from build123d import *

# Parameters (mm, degrees)
ESQUISSE1_W        = 45
ESQUISSE1_H        = 36
BOSS_EXTRU_1_DEPTH = 8
ESQUISSE2_W        = 10.16
ESQUISSE2_H        = 7.62
BOSS_EXTRU_2_DEPTH = 6
ESQUISSE3_R        = 1
BOSS_EXTRU_3_DEPTH = 15
ESQUISSE4_R        = 1
BOSS_EXTRU_4_DEPTH = 15


with BuildPart() as part:
    # Esquisse1 → Boss.-Extru.1 (new body)
    with BuildSketch(Plane(origin=(0, 0, 0), x_dir=(1, 0, 0), z_dir=(0, 1, 0))):
        Rectangle(ESQUISSE1_W, ESQUISSE1_H)
    extrude(amount=BOSS_EXTRU_1_DEPTH)

    # Esquisse2 → Boss.-Extru.2 (add)
    with BuildSketch(Plane.ZY.offset(22.5)):
        with Locations((6.482241764, 4)):
            Rectangle(ESQUISSE2_W, ESQUISSE2_H)
    extrude(amount=BOSS_EXTRU_2_DEPTH)

    # Esquisse3 → Boss.-Extru.3 (add)
    with BuildSketch(Plane.ZY.offset(22.5)):
        with Locations(Location((15.846041743, 6, 0), (0, 0, 180))):
            Circle(ESQUISSE3_R)
        with Locations(Location((15.846041743, 2, 0), (0, 0, 180))):
            Circle(ESQUISSE3_R)
    extrude(amount=BOSS_EXTRU_3_DEPTH)

    # Esquisse4 → Boss.-Extru.4 (add)
    with BuildSketch(Plane(origin=(22.5, 0, 0), x_dir=(0, 0, -1), z_dir=(1, 0, 0))):
        with Locations(Location((-16.5, 5.5, 0), (0, 0, 180))):
            Circle(ESQUISSE4_R)
        with Locations(Location((-16.5, 2.5, 0), (0, 0, 180))):
            Circle(ESQUISSE4_R)
        with Locations(Location((-13.5, 2.5, 0), (0, 0, 180))):
            Circle(ESQUISSE4_R)
        with Locations(Location((-13.5, 5.5, 0), (0, 0, 180))):
            Circle(ESQUISSE4_R)
    extrude(amount=BOSS_EXTRU_4_DEPTH)


solid = part.part
Can you work these out from the model? Positions are in its coordinate system, mm. A direction names the side the tool comes from. Give positions to 0.01 mm unless a question says otherwise; leave off trailing zeros. Loops run counter-clockwise (first coordinate to the right, second up) from the corner with the lowest first, then second, coordinate; pieces in that order, holes last. Notation, with made-up numbers: (29, -25.75) -> (67, -25.75) arc R25 cw to (67, 11.25) -> close; hole circle Ø8 at (71, 34.25). An arc over 180 degrees is marked (long way). Use one line per item in the form item = value.
1) For faces 1 (the face through (-28.5, 4, 6)), 2 (the face through (-25, 0.19, 6)), 3 (the face through (-29.895, 5.7, 14.892)), which set-ups out of +Z, -Z, +X, -X, +Y, -Y let a thin tool reach every point of the face, with its end or its side?
Answers:
face_1 = -Z, -X, +Y, -Y
face_2 = +Z, -Z, -X, -Y
face_3 = -X
2) I need wall thicknesses on line 1 along X through (y, z) = (1.25, 3); line 2 along X through (y, z) = (4, -16); line 3 along Z through (x, y) = (-30, 2.5). Which ranges of each line are inside material? Lowest first, please.
Answers:
line_1 = -28.5 to 22.5
line_2 = -22.5 to 22.5
line_3 = 14.98 to 16.71
3) We'd pull the mould along Y, two halves only. Please class faces 4 (the face through (-25, 7.81, 6)), 5 (the face through (29.895, 2.2, 14.454)), 6 (the face through (29.895, 5.2, 14.454)), 7 (the face through (-37.5, 2, 16)): released by +Y, released by -Y, zero draft, split by the parting line, or undercut.
Answers:
face_4 = released by +Y
face_5 = undercut
face_6 = undercut
face_7 = zero draft
4) If we section it at C-C (x = -31): Please give me the cut outline in (y, z).
Answers:
outline = circle Ø2 at (2, 15.85); circle Ø2 at (6, 15.85)
5) Will these pins go through, and if not, where does the flat tip stop? pin 1 (1.8 mm diameter, centred on x = -26, z = 8.5, fed in from -Y); pin 2 (3 mm diameter, centred on y = 6, z = -9.5, fed in from -X); pin 3 (1.8 mm diameter, centred on x = -25, z = 6.5, fed in from +Y); pin 4 (4 mm diameter, centred on x = 8.5, z = 6, fed in from -Y).
Answers:
pin_1 = 0.19
pin_2 = -22.5
pin_3 = 7.81
pin_4 = 0
6) If we section it at B-B (x = 24.5): Please give me the cut outline in (y, z).
Answers:
outline = circle Ø2 at (2.5, 13.5); circle Ø2 at (2.5, 16.5); circle Ø2 at (5.5, 13.5); circle Ø2 at (5.5, 16.5)
7) If we section it at A-A (z = 10): Please give me the cut outline in (x, y), plus the area to 3 significant figures.
Answers:
outline = (-28.5, 0.19) -> (-22.5, 0.19) -> (-22.5, 0) -> (22.5, 0) -> (22.5, 8) -> (-22.5, 8) -> (-22.5, 7.81) -> (-28.5, 7.81) -> close
area = 406 mm²
